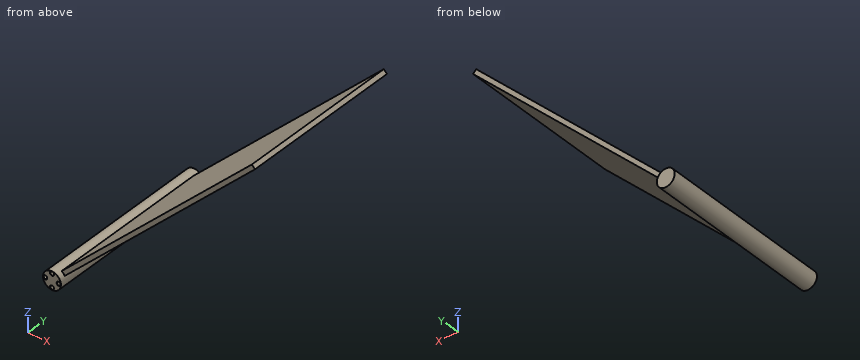
Autodesk Inventor part; units mm, degrees
ref_plane "РабПлоскость1" through (0, 0, 0) normal (0.7071, 0, -0.7071) x (0, 1, 0)
ref_plane "РабПлоскость2" through (7.0711, 0, 7.0711) normal (0.7071, 0, 0.7071) x (0, 1, 0)
ref_plane "XZ Plane" through (0, 0, 0) normal (0, 1, 0) x (-1, 0, 0)
sketch "Эскиз1" plane through (0, 0, 0) normal (0, 1, 0) x (-1, 0, 0)
  circle A0 centre (0, 0) radius 10
  dimension "d0" = 20
extrude "Выдавливание1" add sketch "Эскиз1" along normal blind 194.4
sketch "Эскиз2" plane through (0, 0, 0) normal (0, -1, 0) x (1, 0, 0)
  circle A0 centre (0, 0) radius 7.5 construction
  point P0 (0, 7.5)
  dimension "d3" = 15
hole "Отверстие1" at (0, 0, 7.5) direction (0, 1, 0) diameter 3.9 depth 6 countersink diameter 4.5 countersink angle 90
pattern_circular "Круговой массив1" count 4 over 360 about axis through (0, 0, 0) along (0, 1, 0) of "Отверстие1"
ref_plane "РабПлоскость1" through (0, 0, 0) normal (0.7071, 0, -0.7071) x (0, 1, 0)
sketch "Эскиз3" plane through (0, 0, 0) normal (0.7071, 0, -0.7071) x (0, 1, 0)
  line L0 (0, 10) -> (194.4, 10)
  point P0 (0, 0)
ref_plane "РабПлоскость2" through (7.0711, 0, 7.0711) normal (0.7071, 0, 0.7071) x (0, 1, 0)
sketch "Эскиз4" plane through (7.0711, 0, 7.0711) normal (0.7071, 0, 0.7071) x (0, 1, 0)
  line L0 (6, 3.3533) -> (0.3, 3.3533)
  line L1 (6, 7.2533) -> (0.3, 7.2533)
  line L2 (6, 7.2533) -> (6, 3.3533)
  line L3 (6, -7.2533) -> (0.3, -7.2533)
  line L4 (6, -3.3533) -> (0.3, -3.3533)
  line L5 (6, -3.3533) -> (6, -7.2533)
  line L6 (7, 2.5) -> (187.4, 2.5)
  line L7 (187.4, 2.5) -> (187.4, -2.5)
  line L8 (187.4, -2.5) -> (7, -2.5)
  line L9 (7, -2.5) -> (7, 2.5)
  line L10 (0, 0) -> (8, 0) construction
  line L11 (194.4, -10) -> (194.4, 10) construction
  dimension "d14" = 5
  dimension "d15" = 7
  dimension "d16" = 7
extrude "Выдавливание2" add sketch "Эскиз4" along normal blind 300 and the other way blind 10
properties part number "вал"
Design review of the part built by this model. Coordinates are the model's own, in mm. Coordinates: 2 decimals unless noted, no trailing zeros. Loops run counter-clockwise (first coordinate to the right, second up) from the corner with the lowest first, then second, coordinate; pieces in that order, holes last. Notation, with made-up numbers: (9, 38) - (55, 38) arc R22 ccw to (55, 48) - close; hole circle Ø1 at (-39.75, -34.5). An arc over 180 degrees is marked (long way). Use CSV: the item, a comma, the result in double quotes. Start each with the question number.
1. Add section B-B on z = 115.5. Give the boundary of the cut face in (x, y).
2. Add section A-A on y = 175. Give the boundary of the cut face in (x, z), plus the area to 3 significant figures.
3. To check wall thickness, follow probe 1 along X at (y, z) = (1.75, -7.5); probe 2 along Z at (x, y) = (-7, 4); probe 3 along X at (y, z) = (117.5, 133). State the ranges of each line that lie inside material, in increasing order.
4. Clearance check with flat-ended pins moving along their axes: pin 1 (10 mm diameter, centred on x = 135, y = 21, fed in from +Z); pin 2 (1.2 mm diameter, centred on x = 8.5, z = 0.5, fed in from -Y); pin 3 (4 mm diameter, centred on y = 26.5, z = 138.5, fed in from -X). State where each tip first meets the part, or that it passes through.
Resolved:
1,outline,"(111.96, 7) - (119.04, 7) - (119.04, 187.4) - (111.96, 187.4) - close"
2,outline,"(5.08, 8.61) arc R10 ccw (long way) to (8.61, 5.08) - (220.97, 217.44) - (217.44, 220.97) - close"
2,area,"1,810 mm2"
3,probe 1,"-6.61 to -1.95, 1.95 to 6.61"
3,probe 2,"-7.14 to -1.88, 1.88 to 7.14"
3,probe 3,"129.46 to 136.54"
4,pin 1,"z = 143.54"
4,pin 2,"y = 6"
4,pin 3,"x = 132.96"
